The drawing under review shows one solid part. Ordinate dimensions are in mm from its lowest x, y, z. Coordinates: 2 decimals unless noted, no trailing zeros. Order: outer loops, then holes, each group sorted by start corner. A loop starts at its lowest first (then second) coordinate and runs counter-clockwise, first axis right, second up. Notation, with made-up numbers: M 42,-26 L 93,-26 A6 ccw 93,-16 Z; hole C -1,13.5 d3. An arc over 180 degrees is marked long. Answer as a JSON object with one key per item and string values.
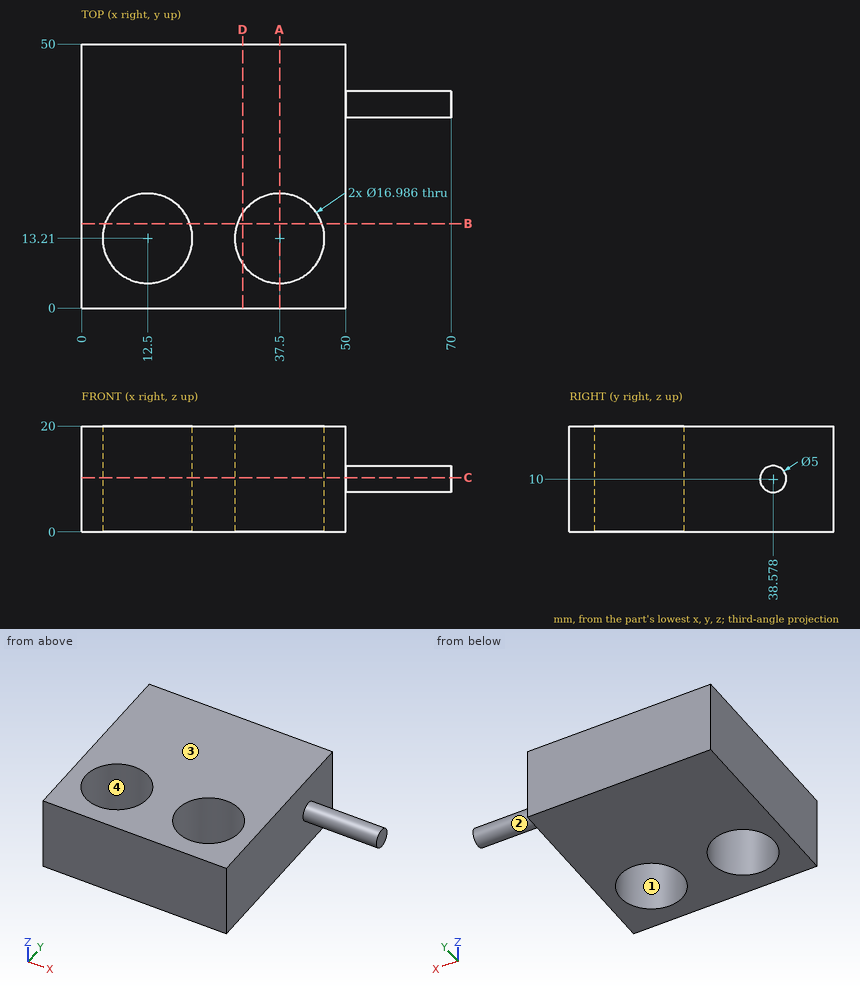
1) Insertion check: pin 1 Ø6 at (y, z) = (43, 15.5) entering from +X; pin 2 Ø10 at (x, y) = (12.5, 13.21) entering from +Z. Each pin has a flat end and moves straight along its axis. Give the tip position at first contact, or say it passes through.
Taken from the geometry:
{"pin 1": "stops at x = 50", "pin 2": "passes through"}
2) Add section C-C (z = 10.25). State the section outline as (x, y) points (1 decimal), and give its area (3 significant figures).
Taken from the geometry:
{"outline": "M 0,0 L 50,0 L 50,36.1 L 70,36.1 L 70,41.1 L 50,41.1 L 50,50 L 0,50 Z; hole C 12.5,13.2 d17; hole C 37.5,13.2 d17", "area": "2,150 mm2"}
3) Add section A-A (x = 37.5). State the section outline as (y, z) points, and give its area (3 significant figures).
Taken from the geometry:
{"outline": "M 0,0 L 4.72,0 L 4.72,20 L 0,20 Z; M 21.7,0 L 50,0 L 50,20 L 21.7,20 Z", "area": "660 mm2"}
4) Mouldability with a two-part tool opening along Y and no side actions: class the marked faces 1, 2, 3 and 4 as released by +Y, released by -Y, zero draft, split by the parting line, or undercut.
Taken from the geometry:
{"face 1": "undercut", "face 2": "split by the parting line", "face 3": "zero draft", "face 4": "undercut"}
5) Add section D-D (x = 30.5). State the section outline as (y, z) points.
Taken from the geometry:
{"outline": "M 0,0 L 8.4,0 L 8.4,20 L 0,20 Z; M 18.02,0 L 50,0 L 50,20 L 18.02,20 Z"}
6) Add section B-B (y = 16). State the section outline as (x, z) points, and give its area (3 significant figures).
Taken from the geometry:
{"outline": "M 0,0 L 4.48,0 L 4.48,20 L 0,20 Z; M 20.52,0 L 29.48,0 L 29.48,20 L 20.52,20 Z; M 45.52,0 L 50,0 L 50,20 L 45.52,20 Z", "area": "358 mm2"}
7) To check wall thickness, follow L1, parallel to X at y = 11.5, z = 11.25; L2, parallel to Y at x = 37.5, z = 10.25; L3, parallel to X at y = 29.5, z = 10. State the ranges of each line that lie inside material, in increasing order.
Taken from the geometry:
{"L1": "x = 0 to 4.18, 20.82 to 29.18, 45.82 to 50", "L2": "y = 0 to 4.72, 21.7 to 50", "L3": "x = 0 to 50"}
